```python
from build123d import *

# Parameters (mm, degrees)
SKETCH1_W            = 29.5
SKETCH1_H            = 6.75
BOSS_EXTRUDE10_DEPTH = 3.5
SKETCH1_16_R         = 0.291434634
BOSS_EXTRUDE15_DEPTH = 1.25
SKETCH1_17_W         = 34.75
SKETCH1_17_H         = 2.924143722
BOSS_EXTRUDE17_DEPTH = 29.25
SKETCH2_W            = 21.15
SKETCH2_H            = 5
BOSS_EXTRUDE18_DEPTH = 1.25
FILLET1_R            = 2
FILLET2_R            = 4
CUT_EXTRUDE1_START   = -2.25
SKETCH3_W            = 5.75
SKETCH3_H            = 1.125
CUT_EXTRUDE1_DEPTH   = 2.25
SKETCH4_R            = 1.75
BOSS_EXTRUDE19_DEPTH = 1.5


with BuildPart() as part:
    # Sketch1 → Boss-Extrude10 (new body)
    with BuildSketch(Plane.XY):
        with Locations((0, 3.375)):
            Rectangle(SKETCH1_W, SKETCH1_H)
        with BuildLine():
            Line((-12.265078429, 5.016721387), (0, 6.25))
            Line((0, 6.25), (12.265078429, 5.016721387))
            ThreePointArc((12.265078429, 5.016721387), (13.75, 3.375), (12.265078429, 1.733278613))
            Line((12.265078429, 1.733278613), (0, 0.5))
            Line((0, 0.5), (-12.265078429, 1.733278613))
            ThreePointArc((-12.265078429, 1.733278613), (-13.75, 3.375), (-12.265078429, 5.016721387))
        make_face(mode=Mode.SUBTRACT)
    extrude(amount=BOSS_EXTRUDE10_DEPTH)

    # Sketch1<16> → Boss-Extrude15 (add)
    # profile 1 of 9: a face of its own
    with BuildSketch(Plane.XY):
        with BuildLine():
            Line((-0.57238697, 6.192445325), (-12.265078429, 5.016721387))
            ThreePointArc((-12.265078429, 5.016721387), (-13.75, 3.375), (-12.265078429, 1.733278613))
            Line((-12.265078429, 1.733278613), (-0.57238697, 0.557554675))
            ThreePointArc((-0.57238697, 0.557554675), (-2.875, 3.375), (-0.57238697, 6.192445325))
        make_face()
        with Locations((-12.1, 3.375)):
            Circle(SKETCH1_16_R, mode=Mode.SUBTRACT)
        with Locations((-10.063185408, 3.375)):
            Circle(SKETCH1_16_R, mode=Mode.SUBTRACT)
        with Locations((-8.026370816, 3.375)):
            Circle(SKETCH1_16_R, mode=Mode.SUBTRACT)
    # profile 2 of 9: a face of its own
    with BuildSketch(Plane.XY):
        with Locations((-12.1, 3.375)):
            Circle(SKETCH1_16_R)
    # profile 3 of 9: a face of its own
    with BuildSketch(Plane.XY):
        with Locations((-8.026370816, 3.375)):
            Circle(SKETCH1_16_R)
    # profile 4 of 9: a face of its own
    with BuildSketch(Plane.XY):
        with Locations((-10.063185408, 3.375)):
            Circle(SKETCH1_16_R)
    # profile 5 of 9: a face of its own
    with BuildSketch(Plane.XY):
        with BuildLine():
            Line((0, 6.25), (-0.57238697, 6.192445325))
            ThreePointArc((-0.57238697, 6.192445325), (-2.875, 3.375), (-0.57238697, 0.557554675))
            Line((-0.57238697, 0.557554675), (0, 0.5))
            Line((0, 0.5), (0.57238697, 0.557554675))
            ThreePointArc((0.57238697, 0.557554675), (2.226121912, 1.555657748), (2.875, 3.375))
            ThreePointArc((2.875, 3.375), (2.226121912, 5.194342252), (0.57238697, 6.192445325))
            Line((0.57238697, 6.192445325), (0, 6.25))
        make_face()
    # profile 6 of 9: a face of its own
    with BuildSketch(Plane.XY):
        with BuildLine():
            Line((12.265078429, 5.016721387), (0.57238697, 6.192445325))
            ThreePointArc((0.57238697, 6.192445325), (2.226121912, 5.194342252), (2.875, 3.375))
            ThreePointArc((2.875, 3.375), (2.226121912, 1.555657748), (0.57238697, 0.557554675))
            Line((0.57238697, 0.557554675), (12.265078429, 1.733278613))
            ThreePointArc((12.265078429, 1.733278613), (13.75, 3.375), (12.265078429, 5.016721387))
        make_face()
        with Locations((8.026370816, 3.375)):
            Circle(SKETCH1_16_R, mode=Mode.SUBTRACT)
        with Locations((10.063185408, 3.375)):
            Circle(SKETCH1_16_R, mode=Mode.SUBTRACT)
        with Locations((12.1, 3.375)):
            Circle(SKETCH1_16_R, mode=Mode.SUBTRACT)
    # profile 7 of 9: a face of its own
    with BuildSketch(Plane.XY):
        with Locations((12.1, 3.375)):
            Circle(SKETCH1_16_R)
    # profile 8 of 9: a face of its own
    with BuildSketch(Plane.XY):
        with Locations((10.063185408, 3.375)):
            Circle(SKETCH1_16_R)
    # profile 9 of 9: a face of its own
    with BuildSketch(Plane.XY):
        with Locations((8.026370816, 3.375)):
            Circle(SKETCH1_16_R)
    extrude(amount=BOSS_EXTRUDE15_DEPTH)

    # Sketch1<17> → Boss-Extrude17 (add)
    with BuildSketch(Plane.XY):
        with Locations((32.125, 3.375)):
            Rectangle(SKETCH1_17_W, SKETCH1_17_H)
    extrude(amount=BOSS_EXTRUDE17_DEPTH)

    # Sketch2 → Boss-Extrude18 (add)
    with BuildSketch(Plane.XY.offset(29.25)):
        with Locations((4.175, 3.375)):
            Rectangle(SKETCH2_W, SKETCH2_H)
    extrude(amount=-BOSS_EXTRUDE18_DEPTH)

    # Fillet1
    # the kernel refuses this fillet: 2 mm, written as the material it adds along each edge
    with BuildSketch(Plane(origin=(14.75, 1.912928139, 0), x_dir=(0, -1, 0), z_dir=(0, 0, 1))) as fillet1_piece_1:
        with BuildLine():
            CenterArc((2, 1.998103724), FILLET1_R, 180, 87.504786267)
            Line((0, 1.998103724), (0, 0))
            Line((0, 0), (1.912928139, 0))
        make_face()
    extrude(amount=3.5)
    with BuildSketch(Plane(origin=(14.75, 4.837071861, 0), x_dir=(1, 0, 0), z_dir=(0, 0, 1))) as fillet1_piece_2:
        with BuildLine():
            CenterArc((1.998103724, 2), FILLET1_R, 182.495213733, 87.504786267)
            Line((0, 1.912928139), (0, 0))
            Line((0, 0), (1.998103724, 0))
        make_face()
    extrude(amount=3.5)
    with BuildSketch(Plane(origin=(14.75, 4.837071861, 28), x_dir=(1, 0, 0), z_dir=(0, 0, 1))) as fillet1_piece_3:
        with BuildLine():
            CenterArc((1.753401761, 2), FILLET1_R, 208.753082152, 61.246917848)
            Line((0, 1.037928139), (0, 0))
            Line((0, 0), (1.753401761, 0))
        make_face()
    extrude(amount=1.25)
    with BuildSketch(Plane(origin=(14.75, 1.912928139, 28), x_dir=(1, 0, 0), z_dir=(0, 0, 1))) as fillet1_piece_4:
        with BuildLine():
            CenterArc((1.753401761, -2), FILLET1_R, 90, 61.246917848)
            Line((0, -1.037928139), (0, 0))
            Line((0, 0), (1.753401761, 0))
        make_face()
    extrude(amount=1.25)

    # Fillet2
    # the kernel refuses this fillet: 4 mm, written as the material it takes off along each edge
    with BuildSketch(Plane(origin=(-14.75, 6.75, -10), x_dir=(0, -1, 0), z_dir=(0, 0, 1)), Plane(origin=(-14.75, 0, -10), x_dir=(1, 0, 0), z_dir=(0, 0, 1))) as fillet2_piece_1:
        with BuildLine():
            CenterArc((FILLET2_R, FILLET2_R), FILLET2_R, 180, 90)
            Line((0, FILLET2_R), (0, 0))
            Line((0, 0), (FILLET2_R, 0))
        make_face()
    extrude(amount=23.5, mode=Mode.SUBTRACT)

    # Sketch3 → Cut-Extrude1 (cut)
    with BuildSketch(Plane.XY.offset(3.5).offset(CUT_EXTRUDE1_START)):
        with Locations((-0.102107464, 6.1875)):
            Rectangle(SKETCH3_W, SKETCH3_H)
        with Locations((-0.102107464, 0.5625)):
            Rectangle(SKETCH3_W, SKETCH3_H)
    extrude(amount=CUT_EXTRUDE1_DEPTH, mode=Mode.SUBTRACT)

    # Sketch4 → Boss-Extrude19 (add)
    with BuildSketch(Plane.XY.offset(29.25)):
        with Locations((0.102107464, 3.375)):
            Circle(SKETCH4_R)
    extrude(amount=BOSS_EXTRUDE19_DEPTH)


solid = part.part
```
The listing builds one solid part. Answer for the finished solid, in the listing's coordinates (mm). A direction names the side the tool comes from. Coordinates: 2 decimals unless noted, no trailing zeros. Loops run counter-clockwise (first coordinate to the right, second up) from the corner with the lowest first, then second, coordinate; pieces in that order, holes last. Notation, with made-up numbers: (81.25, 67.25) -> (130.25, 67.25) arc R26 ccw to (130.25, 86.25) -> close; hole circle Ø8 at (69.5, 76.25). An arc over 180 degrees is marked (long way). Use one line per item in the form item = value. Start each with the question number.
Item 1: The part is cut by section D-D on y = 4. Determine the outline of the cut face in (x, z), then the cut area to 3 significant figures.
Item 2: The part is cut by section C-C on z = 21. Determine the outline of the cut face in (x, y).
Item 3: The mould has two halves that part along Y. Classify faces 6 (the face through (-13.75, 3.34, 2.36)), 7 (the face through (2, 0, 1)), 8 (the face through (-13.318, 5.817, 1.726)): released by +Y, released by -Y, zero draft, split by the parting line, or undercut.
Item 4: Flat-ended cylindrical pins translate along their axes: pin 1 Ø2 at (x, z) = (19.5, 16) entering from -Y; pin 2 Ø3 at (x, y) = (19, 2.5) entering from +Z; pin 3 Ø5 at (x, z) = (-4.5, 4) entering from +Y; pin 4 Ø0.6 at (y, z) = (6.5, 2.5) entering from +X. Find the tip coordinate at first contact, or state that the pin passes through.
Item 5: The part is cut by section A-A on x = 0. Determine the outline of the cut face in (y, z) (3 decimals).
Item 6: The part is cut by section B-B on x = 31. Determine the outline of the cut face in (y, z).
Item 7: Consider L1, parallel to Z at x = 1, y = 1.5; L2, parallel to X at y = 3.5, z = 19.5; L3, parallel to Y at x = 28, z = 10.5. Determine where each line is inside the solid, lowest interval first. Write a range as [from, to].
Item 8: A tool of negligible diameter and unlimited length cuts with its end or side. For faces 1 (the face through (-6.4, 3, 29)), 2 (the face through (4, 0.875, 29)), 3 (the face through (13.75, 3.41, 2.36)), 4 (the face through (14.75, 3, 16)), 5 (the face through (15.472, 5.124, 28.616)), from which of +Z, -Z, +X, -X, +Y, -Y can it reach the whole face along a straight path? Write none if from no direction.
Answer key:
q1.outline = (-14.55, 0) -> (49.5, 0) -> (49.5, 29.25) -> (1.74, 29.25) -> (1.74, 30.75) -> (-1.53, 30.75) -> (-1.53, 29.25) -> (-6.4, 29.25) -> (-6.4, 28) -> (14.75, 28) -> (14.75, 3.5) -> (13.63, 3.5) -> (13.63, 1.25) -> (-13.63, 1.25) -> (-13.63, 3.5) -> (-14.55, 3.5) -> close
q1.area = 1,090 mm2
q2.outline = (14.75, 1.91) -> (49.5, 1.91) -> (49.5, 4.84) -> (14.75, 4.84) -> close
q3.face_6 = undercut
q3.face_7 = released by -Y
q3.face_8 = released by +Y
q4.pin_1 = 1.91
q4.pin_2 = 29.25
q4.pin_3 = 6.75
q4.pin_4 = 14.85
q5.outline = (0, 0) -> (6.75, 0) -> (6.75, 1.25) -> (0, 1.25) -> close; (0.875, 28) -> (5.875, 28) -> (5.875, 29.25) -> (5.122, 29.25) -> (5.122, 30.75) -> (1.628, 30.75) -> (1.628, 29.25) -> (0.875, 29.25) -> close
q6.outline = (1.91, 0) -> (4.84, 0) -> (4.84, 29.25) -> (1.91, 29.25) -> close
q7.L1 = [0, 1.25], [28, 29.25]
q7.L2 = [14.75, 49.5]
q7.L3 = [1.91, 4.84]
q8.face_1 = +Z, -X, +Y, -Y
q8.face_2 = +Z, +X, -X, -Y
q8.face_3 = none
q8.face_4 = -X, +Y, -Y
q8.face_5 = +Z, +X, +Y
